Source: CAD feature listing. Evaluate the final solid. Frame: model axes, mm. Face numbers are marked on the shaded views. A direction names the side the tool comes from. Give positions to 0.01 mm unless a question says otherwise; leave off trailing zeros. Write each loop counter-clockwise with the first axis right and the second up, starting at its lowest first coordinate (ties: lowest second). Pieces come first, ordered by that corner, then holes. Notation, with made-up numbers: M 16,41 L 27,41 A30 ccw 27,70 Z; hole C 28,-15 d9. An arc over 180 degrees is marked long. Answer as a JSON object with one key per item and string values. Group by question number.
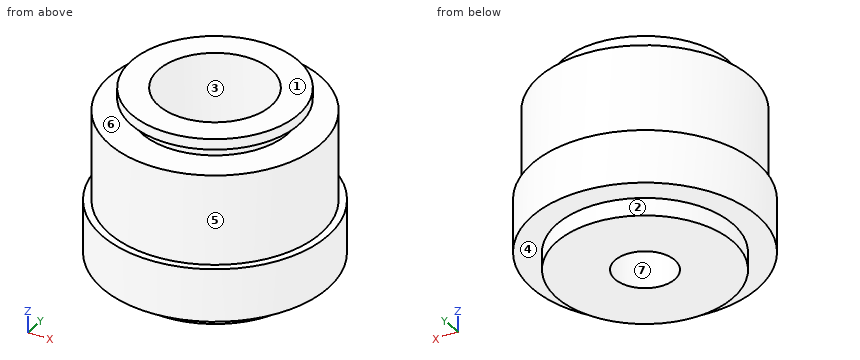
Autodesk Inventor part; units mm, degrees
ref_plane "YZ Plane" through (0, 0, 0) normal (1, 0, 0) x (0, 1, 0)
ref_plane "XZ Plane" through (0, 0, 0) normal (0, 1, 0) x (-1, 0, 0)
ref_plane "XY Plane" through (0, 0, 0) normal (0, 0, 1) x (1, 0, 0)
sketch "Sketch1" plane through (0, 0, 0) normal (0, 1, 0) x (-1, 0, 0)
  line L0 (1.7, -10.4) -> (5, -10.4)
  line L1 (5, -10.4) -> (5, -9.4)
  line L2 (3.2, -7.41) -> (1.7, -7.41)
  line L3 (1.7, -7.41) -> (1.7, -10.4)
  line L4 (5, -9.4) -> (6.408, -9.4)
  line L5 (6.408, -9.4) -> (6.408, -6.4)
  line L6 (6.408, -6.4) -> (6, -6.4)
  line L7 (3.2, 0) -> (3.2, -7.41)
  line L8 (3.2, 0) -> (6, 0)
  line L9 (6, 0) -> (6, -6.4)
  line L10 (0, 0) -> (0, -11.6607)
  dimension "d0" = 5
  dimension "d1" = 10.4
  dimension "d2" = 1
  dimension "d3" = 0
  dimension "d4" = 3
  dimension "d5" = 7.41
  dimension "d6" = 1.7
  dimension "d8" = 6
  dimension "d9" = 6.408
  dimension "d10" = 3.2
revolve "Revolution1" add sketch "Sketch1" angle 360 about axis through (0, 0, 0) along (0, 0, -1)
sketch "Sketch3" plane through (0, 0, 0) normal (1, 0, 0) x (0, 1, 0)
  line L0 (1.7, -10.4) -> (1.7, -7.41) construction
  line L1 (1.7, -7.41) -> (3.2, -7.41) construction
  line L2 (3.2, -7.41) -> (3.2, 0) construction
  line L3 (3.2, 0) -> (6, 0) construction
  line L4 (6, 0) -> (6, -6.4) construction
  line L5 (6, -6.4) -> (6.408, -6.4) construction
  line L6 (6.408, -6.4) -> (6.408, -9.4) construction
  line L7 (6.408, -9.4) -> (5, -9.4) construction
  line L8 (5, -9.4) -> (5, -10.4) construction
  line L9 (5, -10.4) -> (1.7, -10.4) construction
  line L10 (-1.7, -7.41) -> (-1.7, -10.4) construction
  line L11 (-1.7, -10.4) -> (-5, -10.4) construction
  line L12 (-5, -10.4) -> (-5, -9.4) construction
  line L13 (-5, -9.4) -> (-6.408, -9.4) construction
  line L14 (-6.408, -9.4) -> (-6.408, -6.4) construction
  line L15 (-6.408, -6.4) -> (-6, -6.4) construction
  line L16 (-6, -6.4) -> (-6, 0) construction
  line L17 (-6, 0) -> (-3.2, 0) construction
  line L18 (-3.2, 0) -> (-3.2, -7.41) construction
  line L19 (-3.2, -7.41) -> (-1.7, -7.41) construction
  line L20 (6, 0) -> (4.15, 0)
  line L21 (4.15, -0.6) -> (4.15, -1.3)
  line L22 (4.15, -1.3) -> (6, -1.3)
  line L23 (6, -1.3) -> (6, 0)
  line L24 (-6, 0) -> (6, 0)
  line L25 (4.15, -0.6) -> (4.75, -0.6)
  line L26 (4.75, -0.6) -> (4.75, 0)
  line L27 (4.75, 0) -> (4.15, 0)
  line L28 (0, -12.48) -> (0, 2.08)
  point P0 (0, 0)
  dimension "d13" = 0.6
  dimension "d14" = 1.3
  dimension "d15" = 4.15
  dimension "d16" = 4.75
revolve "Revolution2" cut sketch "Sketch3" angle 360 about axis through (0, 0, -10) along (0, 0, 1)
properties part number "500-107" material "Steel"
(1) Pull-direction query (X, two-part tool) for the marked faces 1, 2 and 3; classes: pulls with the +X half, pulls with the -X half, needs draft (parallel to the pull), parting line crosses it, or undercut.
(2) Contact query for flat-ended pins moving along their axis: pin 1 Ø3 at (y, z) = (5, -4) entering from +X; pin 2 Ø5 at (x, z) = (-0.5, -1.5) entering from +Y; pin 3 Ø2 at (x, z) = (-4, -9) entering from +Y. Output: stop coordinate, or through.
(3) Ray query, L1, parallel to Y at x = 0, z = -8.3; L2, parallel to Z at x = 2.75, y = 3.5; L3, parallel to Y at x = 0, z = -5. Return the intervals inside material, ascending. Write a range as [from, to].
(4) Section D-D, the plane x = 2.5. Return loops of the section in (y, z), plus the area to 3 significant figures.
(5) Section A-A, the plane x = 0. Return loops of the section in (y, z).
(6) Section C-C, the plane z = -4.75. Return loops of the section in (x, y).
(7) Access query for the marked faces 4, 5, 6 and 7. Directions: +Z, -Z, +X, -X, +Y, -Y. A direction counts if a zero-diameter tool reaches every point of the face in a straight line with its end or side. Return the directions, or none.
Reported:
{
 "1": {"face 1": "needs draft", "face 2": "parting line crosses it", "face 3": "undercut"},
 "2": {"pin 1": "stops at x = 4.87", "pin 2": "stops at y = 6", "pin 3": "stops at y = 5.66"},
 "3": {"L1": "y = [-6.41, -1.7], [1.7, 6.41]", "L2": "z = [-10.4, -1.3], [-0.6, 0]", "L3": "y = [-6, -3.2], [3.2, 6]"},
 "4": {"outline": "M -5.9,-9.4 L -4.33,-9.4 L -4.33,-10.4 L 4.33,-10.4 L 4.33,-9.4 L 5.9,-9.4 L 5.9,-6.4 L 5.45,-6.4 L 5.45,-1.3 L 3.31,-1.3 L 3.31,-0.6 L 4.04,-0.6 L 4.04,0 L 2,0 L 2,-7.41 L -2,-7.41 L -2,0 L -4.04,0 L -4.04,-0.6 L -3.31,-0.6 L -3.31,-1.3 L -5.45,-1.3 L -5.45,-6.4 L -5.9,-6.4 Z", "area": "79.6 mm2"},
 "5": {"outline": "M -6.41,-9.4 L -5,-9.4 L -5,-10.4 L -1.7,-10.4 L -1.7,-7.41 L -3.2,-7.41 L -3.2,0 L -4.75,0 L -4.75,-0.6 L -4.15,-0.6 L -4.15,-1.3 L -6,-1.3 L -6,-6.4 L -6.41,-6.4 Z; M 1.7,-10.4 L 5,-10.4 L 5,-9.4 L 6.41,-9.4 L 6.41,-6.4 L 6,-6.4 L 6,-1.3 L 4.15,-1.3 L 4.15,-0.6 L 4.75,-0.6 L 4.75,0 L 3.2,0 L 3.2,-7.41 L 1.7,-7.41 Z"},
 "6": {"outline": "C 0,0 d12; hole C 0,0 d6.4"},
 "7": {"face 4": "-Z", "face 5": "+Z", "face 6": "none", "face 7": "+Z, -Z"}
}
